Geometry: final body of the model. Coordinates: model frame, mm. A direction names the side the tool comes from. Round coordinates to 2 decimals unless told otherwise and drop trailing zeros. Loops run counter-clockwise (first coordinate to the right, second up) from the corner with the lowest first, then second, coordinate; pieces in that order, holes last. Notation, with made-up numbers: (10.25, 88.25) - (47.25, 88.25) arc R22 ccw to (47.25, 126.25) - close; hole circle Ø8 at (-28.75, 62). An arc over 180 degrees is marked (long way). Answer as a JSON object with one key per item and string values. Group by question number.
Item 1: Section B-B (y = 0). Return the cut outline in (x, z), plus the area to 3 significant figures.
Item 2: First-contact query: pin 1 (6 mm diameter, centred on x = 19.5, y = 28, fed in from +Z); pin 2 (21.5 mm diameter, centred on x = -18, y = -12.5, fed in from +Z); pin 3 (1 mm diameter, centred on x = 33, y = 32.5, fed in from +Z). Flat tips, straight axial feed; report the tip coordinate or a pass-through.
Item 3: Line query: line 1 (X direction, y = 33.25, z = -4.75); line 2 (Y direction, x = 33, z = 234); line 3 (Y direction, x = 0, z = 191). Output: solid intervals per line, ascending.
Item 4: Section C-C (x = -20.5). Return the cut outline in (y, z), plus the area to 3 significant figures.
Item 5: Reachability of faces 5 (the face through (-38, -10, 124)), 6 (the face through (29.8, -35.5, 236.6)), 7 (the face through (1, 1, -27)) from +Z, -Z, +X, -X, +Y, -Y: full face, straight path, thin tool, end or side. Return the list, or none.
Item 6: Draft query along X for faces 1 (the face through (35.47, -1.42, 120.78)), 2 (the face through (-41, -19, 111)), 3 (the face through (1, -41, 111)), 4 (the face through (41, -1, 111)). Return one class per face: released by +X, released by -X, zero draft, split by the parting line, or undercut.
Item 7: Section A-A (x = 0). Return the cut outline in (y, z), plus the area to 3 significant figures.
```python
from build123d import *

# Parameters (mm, degrees)
SKETCH_1_W          = 82
SKETCH_1_H          = 82
SKETCH_1_R          = 35.5
EXTRUDE_1_DEPTH     = 245
SKETCH_2_W          = 82
SKETCH_2_H          = 82
EXTRUDE_2_DEPTH     = 27
SKETCH_3_W          = 8
SKETCH_3_H          = 20
CUT_EXTRUDE_1_DEPTH = 245
SKETCH_4_R          = 4
CUT_EXTRUDE_2_DEPTH = 20
FILLET_2_R          = 3
FILLET_3_R          = 3
FILLET_4_R          = 3
FILLET_5_R          = 3
SKETCH_5_R          = 1.05
CUT_EXTRUDE_3_DEPTH = 10
EXTRUDE_START       = 0.2
SKETCH_6_R          = 1.05
EXTRUDE_3_DEPTH     = 0.2


with BuildPart() as part:
    # 草圖1 → 填料-伸長1 (new body)
    with BuildSketch(Plane.XY):
        Rectangle(SKETCH_1_W, SKETCH_1_H)
        Circle(SKETCH_1_R, mode=Mode.SUBTRACT)
    extrude(amount=EXTRUDE_1_DEPTH)

    # 草圖2 → 填料-伸長2 (add)
    with BuildSketch(Plane(origin=(0, 0, 0), x_dir=(-1, 0, 0), z_dir=(0, 0, -1))):
        Rectangle(SKETCH_2_W, SKETCH_2_H)
    extrude(amount=EXTRUDE_2_DEPTH)

    # 草圖3 → 除料-伸長1 (cut)
    with BuildSketch(Plane.XY.offset(245)):
        with Locations((-37, 0)):
            Rectangle(SKETCH_3_W, SKETCH_3_H)
    extrude(amount=-CUT_EXTRUDE_1_DEPTH, mode=Mode.SUBTRACT)

    # 草圖4 → 除料-伸長2 (cut)
    with BuildSketch(Plane.XY.offset(245)):
        with Locations((-32.9, 33)):
            Circle(SKETCH_4_R)
        with Locations((33.1, 32.9)):
            Circle(SKETCH_4_R)
        with Locations((33, -33.1)):
            Circle(SKETCH_4_R)
        with Locations((-33, -33)):
            Circle(SKETCH_4_R)
    extrude(amount=-CUT_EXTRUDE_2_DEPTH, mode=Mode.SUBTRACT)

    # 圓角2
    fillet_2_edges = [part.edges().sort_by_distance(p)[0] for p in [
        (-36.9, 33, 225),
    ]]
    fillet(fillet_2_edges, radius=FILLET_2_R)

    # 圓角3
    fillet_3_edges = [part.edges().sort_by_distance(p)[0] for p in [
        (29.1, 32.9, 225),
    ]]
    fillet(fillet_3_edges, radius=FILLET_3_R)

    # 圓角4
    fillet_4_edges = [part.edges().sort_by_distance(p)[0] for p in [
        (-37, -33, 225),
    ]]
    fillet(fillet_4_edges, radius=FILLET_4_R)

    # 圓角5
    fillet_5_edges = [part.edges().sort_by_distance(p)[0] for p in [
        (29, -33.1, 225),
    ]]
    fillet(fillet_5_edges, radius=FILLET_5_R)

    # 草圖5 → 除料-伸長3 (cut)
    with BuildSketch(Plane(origin=(0, 41, 0), x_dir=(1, 0, 0), z_dir=(0, 1, 0))):
        with Locations(Location((-36.75, 22.75, 0), (0, 0, 270))):
            Circle(SKETCH_5_R)
        with Locations(Location((-36.75, 4.75, 0), (0, 0, 270))):
            Circle(SKETCH_5_R)
    extrude(amount=-CUT_EXTRUDE_3_DEPTH, mode=Mode.SUBTRACT)

    # 草圖6 → 填料-伸長3 (add)
    with BuildSketch(Plane(origin=(0, 35, 0), x_dir=(1, 0, 0), z_dir=(0, 1, 0)).offset(EXTRUDE_START)):
        with Locations(Location((-36.75, 22.75, 0), (0, 0, 270))):
            Circle(SKETCH_6_R)
        with Locations(Location((-36.75, 4.75, 0), (0, 0, 270))):
            Circle(SKETCH_6_R)
    extrude(amount=-EXTRUDE_3_DEPTH)


solid = part.part
```
Values:
{
 "1": {"outline": "(-41, -27) - (41, -27) - (41, 245) - (35.5, 245) - (35.5, 0) - (-41, 0) - close", "area": "3,560 mm^2"},
 "2": {"pin 1": "stops at z = 245", "pin 2": "stops at z = 0", "pin 3": "stops at z = 225"},
 "3": {"line 1": "x = -41 to -37.8, -35.7 to 41", "line 2": "y = -41 to -37.1, -29.1 to -13.09, 13.09 to 28.9, 36.9 to 41", "line 3": "y = -41 to -35.5, 35.5 to 41"},
 "4": {"outline": "(-41, -27) - (41, -27) - (41, 245) - (28.98, 245) - (28.98, 0) - (-28.98, 0) - (-28.98, 245) - (-41, 245) - close", "area": "8,100 mm^2"},
 "5": {"face 5": "+Z, -X", "face 6": "+Z", "face 7": "-Z, +X, -X, +Y, -Y"},
 "6": {"face 1": "undercut", "face 2": "released by -X", "face 3": "zero draft", "face 4": "released by +X"},
 "7": {"outline": "(-41, -27) - (41, -27) - (41, 245) - (35.5, 245) - (35.5, 0) - (-35.5, 0) - (-35.5, 245) - (-41, 245) - close", "area": "4,910 mm^2"}
}
